Build history of the part. All positions in model axes, mm. Face numbers are marked on the shaded views. A direction names the side the tool comes from. Round coordinates to 2 decimals unless told otherwise and drop trailing zeros. Write each loop counter-clockwise with the first axis right and the second up, starting at its lowest first coordinate (ties: lowest second). Pieces come first, ordered by that corner, then holes.
1) Which spindle directions (+Z, -Z, +X, -X, +Y, -Y) get a long thin tool onto all of the face, cutting with end or side? Do the marked faces 1 and 2. Say none if no direction does.
2) Saw through at A-A (x = 10). Write the cut outline in (y, z), plus the area to 3 significant figures.
3) Saw through at B-B (y = 3.75). Write the cut outline in (x, z).
4) Flat gauge pins, fed straight in: pin 1 (3.5 mm diameter, centred on x = -10, z = -18, fed in from +Y); pin 2 (6 mm diameter, centred on x = -10.5, z = -17.5, fed in from -Y); pin 3 (12 mm diameter, centred on x = -7.5, z = 17.5, fed in from -Y). Where does each tip first touch, or does it go through?
5) Pull direction X, two halves, no side cores. Call the marked faces 3, 4 and 5: +X half, -X half, draft (parallel to the pull), parting line (faces both ways), or undercut.
6) Saw through at C-C (y = -3.5). Write the cut outline in (x, z), plus the area to 3 significant figures.
7) Saw through at D-D (z = 4). Write the cut outline in (x, y).
8) Wall check: probe 1 along X at (y, z) = (0, 18); probe 2 along Z at (x, y) = (10, -6.45); probe 3 along X at (y, z) = (1, 16). Give the ranges that are in metal, low to high.
from build123d import *

# Parameters (mm, degrees)
BOSS_EXTRUDE2_DEPTH = 25
SKETCH2_R           = 2.75
CUT_EXTRUDE1_DEPTH  = 3.5
SKETCH2_3_R         = 2.75
CUT_EXTRUDE2_DEPTH  = 33.787192744


with BuildPart() as part:
    # Sketch1 → Boss-Extrude2 (new, symmetric)
    with BuildSketch(Plane.XY):
        with BuildLine():
            Line((6, 7.5), (15, 7.5))
            Line((15, 7.5), (15, -6.5))
            ThreePointArc((15, -6.5), (14.707106781, -7.207106781), (14, -7.5))
            Line((14, -7.5), (-14, -7.5))
            ThreePointArc((-14, -7.5), (-14.707106781, -7.207106781), (-15, -6.5))
            Line((-15, -6.5), (-15, 7.5))
            Line((-15, 7.5), (-6, 7.5))
            ThreePointArc((-6, 7.5), (0, 1.5), (6, 7.5))
        make_face()
    extrude(amount=BOSS_EXTRUDE2_DEPTH, both=True)

    # Sketch2 → Cut-Extrude1 (cut)
    # profile 1 of 12: a face of its own
    with BuildSketch(Plane.XZ.offset(7.5)):
        with BuildLine():
            Line((-14, 22.631889463), (-14, 13.368110537))
            ThreePointArc((-14, 13.368110537), (-7.453001767, 12.435181944), (-3.88, 18))
            ThreePointArc((-3.88, 18), (-7.453001767, 23.564818056), (-14, 22.631889463))
        make_face()
        with Locations((-10, 18)):
            Circle(SKETCH2_R, mode=Mode.SUBTRACT)
    # profile 2 of 12: a face of its own
    with BuildSketch(Plane.XZ.offset(7.5)):
        with Locations((-10, 18)):
            Circle(SKETCH2_R)
    # profile 3 of 12: a face of its own
    with BuildSketch(Plane.XZ.offset(7.5)):
        with BuildLine():
            Line((14, 13.368110537), (14, 22.631889463))
            ThreePointArc((14, 22.631889463), (3.88, 18), (14, 13.368110537))
        make_face()
        with Locations((10, 18)):
            Circle(SKETCH2_R, mode=Mode.SUBTRACT)
    # profile 4 of 12: a face of its own
    with BuildSketch(Plane.XZ.offset(7.5)):
        with BuildLine():
            ThreePointArc((14, 13.368110537), (15.564818056, 15.453001767), (16.12, 18))
            ThreePointArc((16.12, 18), (15.564818056, 20.546998233), (14, 22.631889463))
            Line((14, 22.631889463), (14, 13.368110537))
        make_face()
    # profile 5 of 12: a face of its own
    with BuildSketch(Plane.XZ.offset(7.5)):
        with BuildLine():
            ThreePointArc((-14, 22.631889463), (-16.12, 18), (-14, 13.368110537))
            Line((-14, 13.368110537), (-14, 22.631889463))
        make_face()
    # profile 6 of 12: a face of its own
    with BuildSketch(Plane.XZ.offset(7.5)):
        with BuildLine():
            ThreePointArc((-14, -22.631889463), (-7.453001767, -23.564818056), (-3.88, -18))
            ThreePointArc((-3.88, -18), (-7.453001767, -12.435181944), (-14, -13.368110537))
            Line((-14, -13.368110537), (-14, -22.631889463))
        make_face()
        with Locations((-10, -18)):
            Circle(SKETCH2_R, mode=Mode.SUBTRACT)
    # profile 7 of 12: a face of its own
    with BuildSketch(Plane.XZ.offset(7.5)):
        with BuildLine():
            Line((-14, -22.631889463), (-14, -13.368110537))
            ThreePointArc((-14, -13.368110537), (-16.12, -18), (-14, -22.631889463))
        make_face()
    # profile 8 of 12: a face of its own
    with BuildSketch(Plane.XZ.offset(7.5)):
        with Locations((-10, -18)):
            Circle(SKETCH2_R)
    # profile 9 of 12: a face of its own
    with BuildSketch(Plane.XZ.offset(7.5)):
        with BuildLine():
            Line((14, -22.631889463), (14, -13.368110537))
            ThreePointArc((14, -13.368110537), (3.88, -18), (14, -22.631889463))
        make_face()
        with Locations((10, -18)):
            Circle(SKETCH2_R, mode=Mode.SUBTRACT)
    # profile 10 of 12: a face of its own
    with BuildSketch(Plane.XZ.offset(7.5)):
        with Locations((10, -18)):
            Circle(SKETCH2_R)
    # profile 11 of 12: a face of its own
    with BuildSketch(Plane.XZ.offset(7.5)):
        with BuildLine():
            ThreePointArc((16.12, -18), (15.564818056, -15.453001767), (14, -13.368110537))
            Line((14, -13.368110537), (14, -22.631889463))
            ThreePointArc((14, -22.631889463), (15.564818056, -20.546998233), (16.12, -18))
        make_face()
    # profile 12 of 12: a face of its own
    with BuildSketch(Plane.XZ.offset(7.5)):
        with Locations((10, 18)):
            Circle(SKETCH2_R)
    extrude(amount=-CUT_EXTRUDE1_DEPTH, mode=Mode.SUBTRACT)

    # Sketch2_3 → Cut-Extrude2 (cut, through all)
    with BuildSketch(Plane.XZ.offset(7.5)):
        with Locations(Location((-10, 18, 0), (0, 0, 270))):
            Circle(SKETCH2_3_R)
        with Locations(Location((10, 18, 0), (0, 0, 270))):
            Circle(SKETCH2_3_R)
        with Locations(Location((10, -18, 0), (0, 0, 270))):
            Circle(SKETCH2_3_R)
        with Locations(Location((-10, -18, 0), (0, 0, 270))):
            Circle(SKETCH2_3_R)
    extrude(amount=-CUT_EXTRUDE2_DEPTH, mode=Mode.SUBTRACT)


solid = part.part
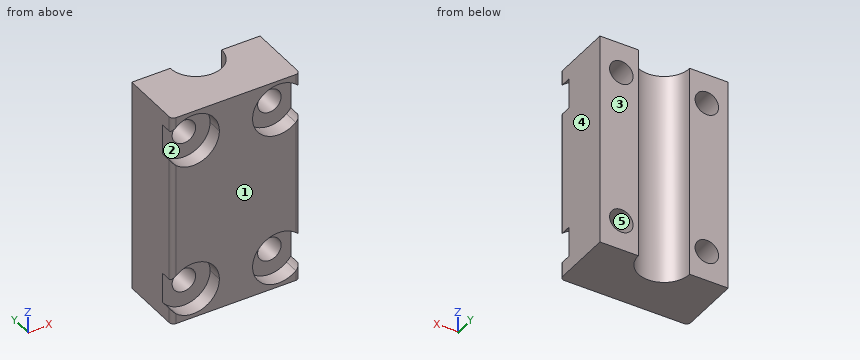
Evaluation:
1. face 1: +Z, -Z, +X, -X, -Y
1. face 2: -Y
2. outline: (-7.5, -25) - (7.5, -25) - (7.5, -20.75) - (-4, -20.75) - (-4, -24.12) - (-7.5, -24.12) - close; (-7.5, -11.88) - (-4, -11.88) - (-4, -15.25) - (7.5, -15.25) - (7.5, 15.25) - (-4, 15.25) - (-4, 11.88) - (-7.5, 11.88) - close; (-7.5, 24.12) - (-4, 24.12) - (-4, 20.75) - (7.5, 20.75) - (7.5, 25) - (-7.5, 25) - close
2. area: 538 mm2
3. outline: (-15, -25) - (-4.68, -25) - (-4.68, 25) - (-15, 25) - close; (4.68, -25) - (15, -25) - (15, 25) - (4.68, 25) - close; hole circle Ø5.5 at (-10, -18); hole circle Ø5.5 at (-10, 18); hole circle Ø5.5 at (10, -18); hole circle Ø5.5 at (10, 18)
4. pin 1: passes through
4. pin 2: stops at y = -4
4. pin 3: stops at y = -7.5
5. face 3: draft
5. face 4: +X half
5. face 5: undercut
6. outline: (-15, -25) - (15, -25) - (15, 25) - (-15, 25) - close; hole circle Ø5.5 at (-10, -18); hole circle Ø5.5 at (-10, 18); hole circle Ø5.5 at (10, -18); hole circle Ø5.5 at (10, 18)
6. area: 1,400 mm2
7. outline: (-15, -6.5) arc R1 ccw to (-14, -7.5) - (14, -7.5) arc R1 ccw to (15, -6.5) - (15, 7.5) - (6, 7.5) arc R6 cw to (-6, 7.5) - (-15, 7.5) - close
8. probe 1: x = -15 to -12.75, -7.25 to 7.25, 12.75 to 15
8. probe 2: z = -25 to -24.12, -11.88 to 11.88, 24.12 to 25
8. probe 3: x = -15 to -11.89, -8.11 to 8.11, 11.89 to 15
